Work out the finished part from the listing and answer in its coordinate system (mm). Face numbers are marked on the shaded views. A direction names the side the tool comes from. Coordinates: 2 decimals unless noted, no trailing zeros. Write each loop counter-clockwise with the first axis right and the second up, starting at its lowest first coordinate (ties: lowest second). Pieces come first, ordered by that corner, then holes. Notation, with made-up numbers: (45.5, 81) - (68.5, 81) arc R34 ccw to (68.5, 118) - close; hole circle Ø1 at (6, -1). An arc over 180 degrees is marked (long way). Use one line per item in the form item = value. Start each with the question number.
Item 1: Given pin 1 (4.5 mm diameter, centred on x = 3.5, z = 3.5, fed in from -Y) (3 decimals); pin 2 (0.7 mm diameter, centred on x = 1, y = -3.5, fed in from +Z); pin 3 (2 mm diameter, centred on x = -7, z = -10.5, fed in from -Y), each flat-ended and moving along its own axis, determine where each tip first touches the part or whether it passes through.
Item 2: A cutting plane is placed at A-A (z = 0). Write down the section's boundary in (x, y) (3 decimals), then the cut area to 3 significant figures.
Item 3: A cutting plane is placed at B-B (z = 4.25). Write down the section's boundary in (x, y) (3 decimals).
Item 4: Consider probe 1 along Z at (x, y) = (0, 0.9) (3 decimals); probe 2 along Y at (x, z) = (-3.75, 4.25) (3 decimals); probe 3 along X at (y, z) = (0, -14). Determine where each line is inside the solid, lowest interval first.
Item 5: For the marked faces 4, 5, 6 and 7, determine the directions among +Z, -Z, +X, -X, +Y, -Y from which every point of the face is accessible in a straight line to the end or side of a thin tool.
Item 6: A cutting plane is placed at C-C (x = -1.25). Give the number of separate pieces and of enclosed holes in the cut face, then the cut area to 3 significant figures.
Item 7: Determine the mould class of the marked faces 1, 2 and 3 for opening direction X: released by +X, released by -X, zero draft, split by the parting line, or undercut.
Item 8: A cutting plane is placed at D-D (y = 4.25). Write down the section's boundary in (x, z).
from build123d import *

# Parameters (mm, degrees)
F0_R     = 8.485
F0_R_2   = 4.675
F1_DEPTH = 2.125
F3_DEPTH = 4.539996
F5_DEPTH = 2.0625
F6_R     = 2.06249
F7_R     = 1.905


# Not quite as in the source:
# - a fillet or chamfer is up to 0.001 mm smaller than in the source, because OpenCascade refuses the exact size


with BuildPart() as f1:
    # F0 (on Front) → F1 (new body, symmetric)
    with BuildSketch(Plane.XZ):
        Circle(F0_R)
        Circle(F0_R_2, mode=Mode.SUBTRACT)
    extrude(amount=F1_DEPTH, both=True)

    # F2 (on Front) → F3 (join, symmetric)
    with BuildSketch(Plane.XZ):
        Polygon((-6.2906053879, -5.6941644561), (-9.7885362858, -18.7486202883), (9.7885362858, -18.7486202883), (6.2906053879, -5.6941644561), align=None)
    extrude(amount=F3_DEPTH, both=True)

    # F4 (on Front) → F5 (cut, symmetric)
    with BuildSketch(Plane.XZ):
        Polygon((4.22592549, -7.8024805709), (0.2414814566, -8.8701091319), (2.8884205433, -18.7486202883), (7.1589347875, -18.7486202883), align=None)
        Polygon((-0.2414814566, -8.8701091319), (-4.22592549, -7.8024805709), (-6.8555269883, -17.6162869659), (-7.1589347875, -18.7486202883), (-2.8884205433, -18.7486202883), align=None)
    extrude(amount=F5_DEPTH, both=True, mode=Mode.SUBTRACT)

    # F6 (radius 2.0625 in the source; OpenCascade refuses exactly that, so slightly less here)
    f6_edges = [f1.edges().sort_by_distance(p)[0] for p in [
        (-5.69243, -2.0625, -13.27555),
        (1.564951, -2.0625, -13.809365),
        (5.69243, -2.0625, -13.27555),
        (-1.564951, -2.0625, -13.809365),
        (5.69243, 2.0625, -13.27555),
        (-1.564951, 2.0625, -13.809365),
        (-5.69243, 2.0625, -13.27555),
        (1.564951, 2.0625, -13.809365),
    ]]
    fillet(f6_edges, radius=F6_R)

    # F7
    f7_edges = [f1.edges().sort_by_distance(p)[0] for p in [
        (8.039571, 4.539996, -12.221392),
        (8.039571, -4.539996, -12.221392),
        (-8.039571, 4.539996, -12.221392),
        (-8.039571, -4.539996, -12.221392),
    ]]
    fillet(f7_edges, radius=F7_R)


solid = f1.part
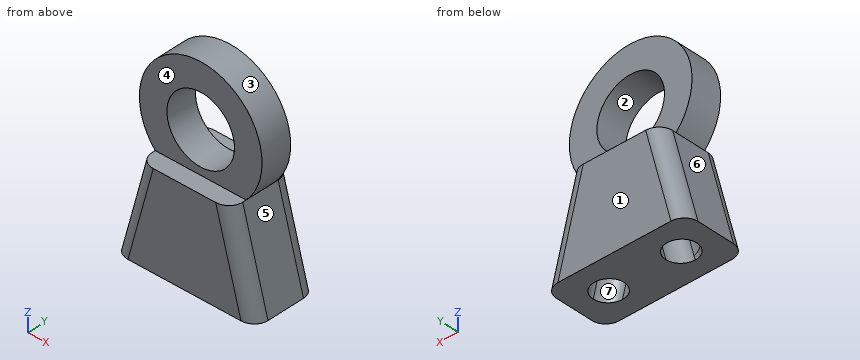
Answer:
q1.pin_1 = -2.125
q1.pin_2 = -5.69
q1.pin_3 = -4.51
q2.outline = (-8.485, -2.125) - (-4.675, -2.125) - (-4.675, 2.125) - (-8.485, 2.125) - close; (4.675, -2.125) - (8.485, -2.125) - (8.485, 2.125) - (4.675, 2.125) - close
q2.area = 32.4 mm²
q3.outline = (-7.344, -2.125) - (-1.948, -2.125) - (-1.948, 2.125) - (-7.344, 2.125) - close; (1.948, -2.125) - (7.344, -2.125) - (7.344, 2.125) - (1.948, 2.125) - close
q4.probe_1 = -18.749 to -4.675, 4.675 to 8.485
q4.probe_2 = -2.125 to 2.125
q4.probe_3 = -8.52 to -5.89, -1.62 to 1.62, 5.89 to 8.52
q5.face_4 = +Z, +X, -X, -Y
q5.face_5 = +X, +Y, -Y
q5.face_6 = -X, +Y, -Y
q5.face_7 = none
q6.separate_pieces = 2
q6.enclosed_holes = 1
q6.area = 130 mm²
q7.face_1 = zero draft
q7.face_2 = undercut
q7.face_3 = split by the parting line
q8.outline = (-8.86, -18.75) - (8.86, -18.75) - (5.36, -5.69) - (-5.36, -5.69) - close
